Design review of the part built by this model. Coordinates are the model's own, in mm. A direction names the side the tool comes from. Coordinates: 2 decimals unless noted, no trailing zeros. Write each loop counter-clockwise with the first axis right and the second up, starting at its lowest first coordinate (ties: lowest second). Pieces come first, ordered by that corner, then holes.
Q1. Machinability: for faces 1 (the cylindrical face through (-48.408, -37.118, -2.465)), 2 (the flat face through (-10.567, 10.646, 0.986)), 3 (the cylindrical face through (-55.55, -42.594, 4.93)), which of the approach directions +Z, -Z, +X, -X, +Y, -Y give a long, thin tool a straight path to every point of the face, cutting with its end or side? Answer none if there is none.
Q2. For probe 1 along X at (y, z) = (2, -0.5); probe 2 along Y at (x, z) = (-4, -18); probe 3 along Y at (x, z) = (34, -5), list the stretches that pass through material, from the lowest coordinate up.
Q3. Take a section at A-A (z = -2.5). Give the boundary of the cut face in (x, y), and give its area (3 significant figures).
Q4. Mouldability with a two-part tool opening along X and no side actions: class faces 4 (the cylindrical face through (0, 2, -26)), 5 (the flat face through (11, -11, -15)), 6 (the flat face through (10.8, 10.8, 0)), 7 (the flat face through (-10.8, 10.8, 0)) as pulls with the +X half, pulls with the -X half, needs draft (parallel to the pull), parting line crosses it, or undercut.
Q5. Insertion check: pin 1 (3 mm diameter, centred on x = -10.5, y = -12, fed in from +Z); pin 2 (3 mm diameter, centred on x = -30, y = 5, fed in from -Z); pin 3 (8 mm diameter, centred on x = 31, z = -17.5, fed in from +Y). Each pin has a flat end and moves straight along its axis. Give the tip position at first contact, or say it passes through.
```python
from build123d import *

# Parameters (mm, degrees)
SKETCH2_R           = 70
BOSS_EXTRUDE2_DEPTH = 10
SKETCH3_R           = 61
BOSS_EXTRUDE3_DEPTH = 15
CUT_EXTRUDE2_DEPTH  = 10
SKETCH10_W          = 15.529142706
SKETCH10_H          = 10
BOSS_EXTRUDE4_DEPTH = 2
SKETCH19_R          = 2
BOSS_EXTRUDE5_DEPTH = 16.7
FILLET1_R           = 10


with BuildPart() as part:
    # Sketch2 → Boss-Extrude2 (new body)
    with BuildSketch(Plane.XY):
        Circle(SKETCH2_R)
    extrude(amount=BOSS_EXTRUDE2_DEPTH)

    # Sketch3 → Boss-Extrude3 (add)
    with BuildSketch(Plane.XY):
        Circle(SKETCH3_R)
    extrude(amount=-BOSS_EXTRUDE3_DEPTH)

    # Sketch9 → Cut-Extrude2 (cut)
    with BuildSketch(Plane.XY.offset(10)):
        Polygon((0, 15.529142706), (-7.764571353, 13.448632083), (-13.448632083, 7.764571353), (-15.529142706, 0), (-13.448632083, -7.764571353), (-7.764571353, -13.448632083), (0, -15.529142706), (7.764571353, -13.448632083), (13.448632083, -7.764571353), (15.529142706, 0), (13.448632083, 7.764571353), (7.764571353, 13.448632083), align=None)
    extrude(amount=-CUT_EXTRUDE2_DEPTH, mode=Mode.SUBTRACT)

    # Sketch10 → Cut-Revolve7 (revolve, cut)
    with BuildSketch(Plane(origin=(0, 0, 0), x_dir=(1, 0, 0), z_dir=(0, 1, 0)), mode=Mode.PRIVATE) as cut_revolve7_sk:
        Polygon((-70, -10), (-15.529142706, -10), (-15.529142706, 0), align=None)
        with Locations((-7.764571353, -5)):
            Rectangle(SKETCH10_W, SKETCH10_H)
    revolve(cut_revolve7_sk.sketch.rotate(Axis((0, 0, 10), (0, 0, -1)), 180), axis=Axis((0, 0, 10), (0, 0, -1)), mode=Mode.SUBTRACT)

    # Sketch14 → Boss-Extrude4 (add)
    with BuildSketch(Plane.XY):
        Polygon((0, 15.529142706), (-7.764571353, 13.448632083), (-13.448632083, 7.764571353), (-15.529142706, 0), (-13.448632083, -7.764571353), (-7.764571353, -13.448632083), (0, -15.529142706), (7.764571353, -13.448632083), (13.448632083, -7.764571353), (15.529142706, 0), (13.448632083, 7.764571353), (7.764571353, 13.448632083), align=None)
    extrude(amount=BOSS_EXTRUDE4_DEPTH)

    # Sketch19 → Boss-Extrude5 (add)
    with BuildSketch(Plane(origin=(0, 0, -15), x_dir=(-1, 0, 0), z_dir=(0, 0, -1))):
        with Locations(Location((0, 0, 0), (0, 0, 180))):
            Circle(SKETCH19_R)
    extrude(amount=BOSS_EXTRUDE5_DEPTH)

    # Sketch22 → Revolve2 (revolve)
    with BuildSketch(Plane(origin=(0, 0, -34.3), x_dir=(-1, 0, 0), z_dir=(0, 0, -1))):
        with BuildLine():
            Line((0, -3.7), (0, 3.7))
            ThreePointArc((0, 3.7), (-3.7, 0), (0, -3.7))
        make_face()
    revolve(axis=Axis((0, -3.7, -34.3), (0, 1, 0)))

    # Fillet1
    fillet1_edges = [part.edges().sort_by_distance(p)[0] for p in [
        (-2, 0, -15),
        (-2, 0, -31.187123517),
        (-61, 0, -15),
    ]]
    fillet(fillet1_edges, radius=FILLET1_R)


solid = part.part
```
Response:
1. face 1: -Z
1. face 2: +Z
1. face 3: +Z, -Z
2. probe 1: x = -60.97 to 60.97
2. probe 2: y = -2.76 to 2.76
2. probe 3: y = -50.65 to 50.65
3. outline: circle Ø122 at (0, 0)
3. area: 11,700 mm2
4. face 4: parting line crosses it
4. face 5: needs draft
4. face 6: undercut
4. face 7: undercut
5. pin 1: stops at z = 2
5. pin 2: stops at z = -15
5. pin 3: stops at y = 47.36
